```python
from build123d import *

# Parameters (mm, degrees)
SKETCH_1_W          = 64
SKETCH_1_H          = 64
EXTRUDE_1_DEPTH     = 22
SHELL_1_T           = -2
SKETCH_2_R          = 25
CUT_EXTRUDE_1_DEPTH = 22
SKETCH_3_R          = 2.05
CUT_EXTRUDE_2_DEPTH = 22


with BuildPart() as part:
    # 草图1 → 凸台-拉伸1 (new body)
    with BuildSketch(Plane(origin=(0, 0, 0), x_dir=(1, 0, 0), z_dir=(0, 1, 0))):
        with Locations((-2.874704492, -9.985815603)):
            Rectangle(SKETCH_1_W, SKETCH_1_H)
    extrude(amount=EXTRUDE_1_DEPTH)

    # 抽壳1
    shell_1_openings = [part.faces().sort_by_distance(p)[0] for p in [
        (-2.874704492, 22, 9.985815603),
    ]]
    offset(amount=SHELL_1_T, openings=shell_1_openings, kind=Kind.INTERSECTION)

    # 草图2 → 切除-拉伸1 (cut)
    with BuildSketch(Plane(origin=(0, 2, 0), x_dir=(1, 0, 0), z_dir=(0, 1, 0))):
        with Locations(Location((-2.874704492, -9.985815603, 0), (0, 0, 270))):
            Circle(SKETCH_2_R)
    extrude(amount=-CUT_EXTRUDE_1_DEPTH, mode=Mode.SUBTRACT)

    # 草图3 → 切除-拉伸2 (cut)
    with BuildSketch(Plane(origin=(0, 2, 0), x_dir=(1, 0, 0), z_dir=(0, 1, 0))):
        with Locations(Location((-27.874704492, 15.014184397, 0), (0, 0, 270))):
            Circle(SKETCH_3_R)
        with Locations(Location((22.125295508, 15.014184397, 0), (0, 0, 270))):
            Circle(SKETCH_3_R)
        with Locations(Location((-27.874704492, -34.985815603, 0), (0, 0, 270))):
            Circle(SKETCH_3_R)
        with Locations(Location((22.125295508, -34.985815603, 0), (0, 0, 270))):
            Circle(SKETCH_3_R)
    extrude(amount=-CUT_EXTRUDE_2_DEPTH, mode=Mode.SUBTRACT)


solid = part.part
```
Model file for the job. Use its own axes, mm. A direction names the side the tool comes from. Coordinates: 2 decimals unless noted, no trailing zeros. Loops run counter-clockwise (first coordinate to the right, second up) from the corner with the lowest first, then second, coordinate; pieces in that order, holes last. Notation, with made-up numbers: (55, 73.25) - (98, 73.25) arc R22 ccw to (98, 86.25) - close; hole circle Ø7 at (-16.5, 29.25). An arc over 180 degrees is marked (long way). Write item = value, one per line. Start each with the question number.
Item 1: Wall check: probe 1 along Z at (x, y) = (-8, 7); probe 2 along Z at (x, y) = (-2, 1.25); probe 3 along X at (y, z) = (10, 7). Give the ranges that are in metal, low to high. Write a range as [from, to].
Item 2: Saw through at A-A, the plane x = 19. List the corners of the cut face in (y, z).
Item 3: Pull direction X, two halves, no side cores. Call faces 1 (the face through (-5, 22, 41)), 2 (the face through (29.125, 11, 10)), 3 (the face through (-32.875, 12, 10)), 4 (the face through (-34.875, 11, 10)): +X half, -X half, draft (parallel to the pull), parting line (faces both ways), or undercut.
Item 4: Drop a flat-ended pin along its axis: pin 1 Ø4.5 at (x, z) = (22.13, -15.01) entering from +Y. Give the stop position or say it passes through.
Item 5: Saw through at B-B, the plane z = 28. List the corners of the cut face in (x, y).
Item 6: 3-axis set-ups, long thin cutter, end or side, ignore diameter. For faces 5 (the face through (-3, 12, 39.986)), 6 (the face through (-26.146, 1.014, -13.912)): which of +Z, -Z, +X, -X, +Y, -Y reach the whole face in a straight line?
Item 7: Saw through at C-C, the plane y = 12.75. List the corners of the cut face in (x, z), then the cut area to 3 significant figures.
Answers:
q1.probe_1 = [-22.01, -20.01], [39.99, 41.99]
q1.probe_2 = [-22.01, -15], [34.97, 41.99]
q1.probe_3 = [-34.87, -32.87], [27.13, 29.13]
q2.outline = (0, -22.01) - (22, -22.01) - (22, -20.01) - (2, -20.01) - (2, -2.12) - (0, -2.12) - close; (0, 22.09) - (2, 22.09) - (2, 39.99) - (22, 39.99) - (22, 41.99) - (0, 41.99) - close
q3.face_1 = draft
q3.face_2 = +X half
q3.face_3 = undercut
q3.face_4 = -X half
q4.pin_1 = 2
q5.outline = (-34.87, 0) - (-20.21, 0) - (-20.21, 2) - (-32.87, 2) - (-32.87, 22) - (-34.87, 22) - close; (14.46, 0) - (29.13, 0) - (29.13, 22) - (27.13, 22) - (27.13, 2) - (14.46, 2) - close
q6.face_5 = +Y
q6.face_6 = +Y, -Y
q7.outline = (-34.87, -22.01) - (29.13, -22.01) - (29.13, 41.99) - (-34.87, 41.99) - close; hole (-32.87, -20.01) - (27.13, -20.01) - (27.13, 39.99) - (-32.87, 39.99) - close
q7.area = 496 mm2
